from build123d import *

# Parameters (mm, degrees)
ESTRUSIONE_ESTRUSIONE1_DEPTH = 0.75


with BuildPart() as part:
    # Schizzo1 → Estrusione-Estrusione1 (new body)
    with BuildSketch(Plane.XY):
        with BuildLine():
            Line((0.713746427, -2.498112495), (0.812636055, -2.844226194))
            ThreePointArc((0.812636055, -2.844226194), (1.087978373, -3.162719515), (1.508964367, -3.158009901))
            ThreePointArc((1.508964367, -3.158009901), (2.5475521, -2.399995479), (3.24232421, -1.318079558))
            ThreePointArc((3.24232421, -1.318079558), (3.221936632, -0.897561146), (2.887600266, -0.641688948))
            Line((2.887600266, -0.641688948), (2.536208379, -0.563601862))
            ThreePointArc((2.536208379, -0.563601862), (2.474583527, -0.521283499), (2.459520601, -0.448060727))
            ThreePointArc((2.459520601, -0.448060727), (2.37991714, 0.765502714), (1.737102314, 1.79790866))
            ThreePointArc((1.737102314, 1.79790866), (1.706652775, 1.866182313), (1.732050808, 1.936491673))
            Line((1.732050808, 1.936491673), (2.645751311, 2.958039892))
            ThreePointArc((2.645751311, 2.958039892), (3.021925983, 3.124694331), (3.395732971, 2.952794878))
            ThreePointArc((3.395732971, 2.952794878), (0, -4.5), (-3.395732971, 2.952794878))
            ThreePointArc((-3.395732971, 2.952794878), (-3.021925983, 3.124694331), (-2.645751311, 2.958039892))
            Line((-2.645751311, 2.958039892), (-1.732050808, 1.936491673))
            ThreePointArc((-1.732050808, 1.936491673), (-1.706652775, 1.866182313), (-1.737102314, 1.79790866))
            ThreePointArc((-1.737102314, 1.79790866), (-2.37991714, 0.765502714), (-2.459520601, -0.448060727))
            ThreePointArc((-2.459520601, -0.448060727), (-2.474583527, -0.521283499), (-2.536208379, -0.563601862))
            Line((-2.536208379, -0.563601862), (-2.887600266, -0.641688948))
            ThreePointArc((-2.887600266, -0.641688948), (-3.221936632, -0.897561146), (-3.24232421, -1.318079558))
            ThreePointArc((-3.24232421, -1.318079558), (-2.5475521, -2.399995479), (-1.508964367, -3.158009901))
            ThreePointArc((-1.508964367, -3.158009901), (-1.087978373, -3.162719515), (-0.812636055, -2.844226194))
            Line((-0.812636055, -2.844226194), (-0.713746427, -2.498112495))
            ThreePointArc((-0.713746427, -2.498112495), (-0.667830724, -2.439119153), (-0.593840416, -2.428446738))
            ThreePointArc((-0.593840416, -2.428446738), (0, -2.5), (0.593840416, -2.428446738))
            ThreePointArc((0.593840416, -2.428446738), (0.667830724, -2.439119153), (0.713746427, -2.498112495))
        make_face()
    extrude(amount=ESTRUSIONE_ESTRUSIONE1_DEPTH)


solid = part.part
Can you work these out from the model? Positions are in its coordinate system, mm. A direction names the side the tool comes from. Give positions to 0.01 mm unless a question says otherwise; leave off trailing zeros. Loops run counter-clockwise (first coordinate to the right, second up) from the corner with the lowest first, then second, coordinate; pieces in that order, holes last. Notation, with made-up numbers: (-8.5, 7.5) -> (24.5, 7.5) arc R17 ccw to (24.5, 17.5) -> close; hole circle Ø11 at (36.25, 76). An arc over 180 degrees is marked (long way). Write item = value, one per line.
1) Suppose I cut it at B-B on x = 3. Write out the boundary of the cut face in (y, z).
Check result:
outline = (-3.35, 0) -> (-1.8, 0) -> (-1.8, 0.75) -> (-3.35, 0.75) -> close; (-0.68, 0) -> (3.12, 0) -> (3.12, 0.75) -> (-0.68, 0.75) -> close
2) Suppose I cut it at D-D on x = 0. Write out the boundary of the cut face in (y, z).
Check result:
outline = (-4.5, 0) -> (-2.5, 0) -> (-2.5, 0.75) -> (-4.5, 0.75) -> close
3) For faces 1 (the flat face through (0, -3, 0.75)), 2 (the cylindrical face through (-2.56, -2.387, 0.37)), 3 (the flat face through (-2.195, 2.454, 0.37)), which set-ups out of +Z, -Z, +X, -X, +Y, -Y let a thin tool reach every point of the face, with its end or its side?
Check result:
face_1 = +Z, +X, -X, +Y, -Y
face_2 = +Z, -Z
face_3 = +Z, -Z, +Y
4) Suppose I cut it at C-C on z = 0.4. Write out the boundary of the cut face in (x, y), then the cut area to 3 significant figures.
Check result:
outline = (-3.4, 2.95) arc R4.5 ccw (long way) to (3.4, 2.95) arc R0.5 ccw to (2.65, 2.96) -> (1.73, 1.94) arc R0.1 ccw to (1.74, 1.8) arc R2.5 cw to (2.46, -0.45) arc R0.1 ccw to (2.54, -0.56) -> (2.89, -0.64) arc R0.5 cw to (3.24, -1.32) arc R3.5 cw to (1.51, -3.16) arc R0.5 cw to (0.81, -2.84) -> (0.71, -2.5) arc R0.1 ccw to (0.59, -2.43) arc R2.5 cw to (-0.59, -2.43) arc R0.1 ccw to (-0.71, -2.5) -> (-0.81, -2.84) arc R0.5 cw to (-1.51, -3.16) arc R3.5 cw to (-3.24, -1.32) arc R0.5 cw to (-2.89, -0.64) -> (-2.54, -0.56) arc R0.1 ccw to (-2.46, -0.45) arc R2.5 cw to (-1.74, 1.8) arc R0.1 ccw to (-1.73, 1.94) -> (-2.65, 2.96) arc R0.5 ccw to start
area = 27.5 mm2
5) Suppose I cut it at A-A on y = 0. Write out the boundary of the cut face in (x, z).
Check result:
outline = (-4.5, 0) -> (-2.5, 0) -> (-2.5, 0.75) -> (-4.5, 0.75) -> close; (2.5, 0) -> (4.5, 0) -> (4.5, 0.75) -> (2.5, 0.75) -> close
6) Thinking about a two-plate mould opening in X: for faces 4 (the cylindrical face through (0.1, -4.5, 0.4)), 5 (the flat face through (2.18, 2.44, 0.37)), 6 (the flat face through (0, -3, 0)), which applies, released by +X, released by -X, zero draft, split by the parting line, or undercut?
Check result:
face_4 = split by the parting line
face_5 = undercut
face_6 = zero draft
7) I need wall thicknesses on L1, parallel to X at y = -2.75, z = 0.7; L2, parallel to X at y = 2.25, z = 0.2; L3, parallel to X at y = -2.25, z = 0.65. Which ranges of each line are inside material? Lowest first, please. Write a range as from..to.
Check result:
L1 = -3.56..-2.17, -0.79..0.79, 2.17..3.56
L2 = -3.9..-2.01, 2.01..3.9
L3 = -3.9..-2.68, 2.68..3.9
